For this review, take the finished solid that the model builds, in its own axes (mm). Face numbers are marked on the shaded views. A direction names the side the tool comes from. Give positions to 0.01 mm unless a question says otherwise; leave off trailing zeros. Write each loop counter-clockwise with the first axis right and the second up, starting at its lowest first coordinate (ties: lowest second). Pieces come first, ordered by that corner, then holes.
1) We need section A-A on z = 23. Give the boundary of the cut face in (x, y).
2) We need section B-B on y = -17. Give the boundary of the cut face in (x, z), and give its area (3 significant figures).
3) Wall thickness on line 1 along Z through (x, y) = (-13.5, 42.5); line 2 along Y through (x, z) = (-95, 29); line 3 along Y through (x, z) = (-90.5, 43): over which ranges is each line inside the solid? List them lowest first.
4) For P1, Ø18.5, axis at x = -77.5, z = 22.5, coming from the +Y side, flat-tipped, find the tip position at first contact; note if it passes through.
5) Machinability: for the marked faces 1, 2 and 3, which of the approach directions +Z, -Z, +X, -X, +Y, -Y give a long, thin tool a straight path to every point of the face, cutting with its end or side? Answer none if there is none.
6) We need section C-C on x = -72. Give the boundary of the cut face in (y, z), and give its area (3 significant figures).
7) We need section D-D on z = 8. Give the boundary of the cut face in (x, y), and give its area (3 significant figures).
from build123d import *

# Parameters (mm, degrees)
F0_W     = 143.607307
F0_H     = 99.53899
F1_DEPTH = 36.83
F2_R     = 15.804954
F3_DEPTH = 25.4
F4_R     = 12.978901
F5_DEPTH = 18.034


with BuildPart() as f1:
    # F0 (on Top) → F1 (new body)
    with BuildSketch(Plane.XY):
        with Locations((-54.842492, 3.94509)):
            Rectangle(F0_W, F0_H)
    extrude(amount=F1_DEPTH)

    # F2 (on face) → F3 (join)
    with BuildSketch(Plane.XY.offset(36.83)):
        with Locations((-90.201773, 32.295499)):
            Circle(F2_R)
    extrude(amount=F3_DEPTH)

    # F4 (on face) → F5 (join)
    with BuildSketch(Plane(origin=(0, 53.714585, 0), x_dir=(-1, 0, 0), z_dir=(0, 1, 0))):
        with Locations((35.902489, 19.206859)):
            Circle(F4_R)
    extrude(amount=F5_DEPTH)


solid = f1.part
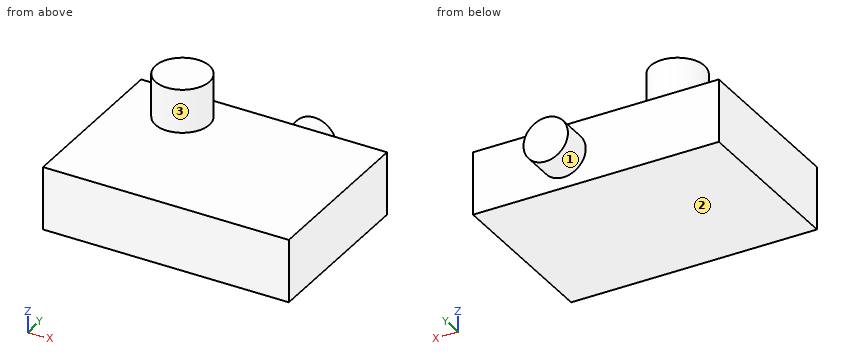
Results list:
1. outline: (-126.65, -45.82) - (16.96, -45.82) - (16.96, 53.71) - (-23.49, 53.71) - (-23.49, 71.75) - (-48.31, 71.75) - (-48.31, 53.71) - (-126.65, 53.71) - close
2. outline: (-126.65, 0) - (16.96, 0) - (16.96, 36.83) - (-126.65, 36.83) - close
2. area: 5,290 mm2
3. line 1: z = 0 to 36.83
3. line 2: y = -45.82 to 53.71
3. line 3: y = 16.49 to 48.1
4. P1: stops at y = 53.71
5. face 1: +Y
5. face 2: -Z, +X, -X, +Y, -Y
5. face 3: +Z
6. outline: (-45.82, 0) - (53.71, 0) - (53.71, 36.83) - (-45.82, 36.83) - close
6. area: 3,670 mm2
7. outline: (-126.65, -45.82) - (16.96, -45.82) - (16.96, 53.71) - (-29.36, 53.71) - (-29.36, 71.75) - (-42.45, 71.75) - (-42.45, 53.71) - (-126.65, 53.71) - close
7. area: 14,500 mm2
